Here's how the part is built. I have some questions about the finished solid (model axes, mm). A direction names the side the tool comes from. Give positions to 0.01 mm unless a question says otherwise; leave off trailing zeros. Loops run counter-clockwise (first coordinate to the right, second up) from the corner with the lowest first, then second, coordinate; pieces in that order, holes last.
Q1. If we section it at B-B (z = -24.5): Please give me the cut outline in (x, y).
Q2. I need wall thicknesses on line 1 (Y direction, x = -8.27, z = 0.2) (3 decimals); line 2 (Z direction, x = 1.5, y = 7.75); line 3 (Y direction, x = 0, z = -28.85). Which ranges of each line are inside material? Lowest first, please.
Q3. If we section it at D-D (x = -8.27): Please give me the cut outline in (y, z) (3 decimals), plus the area to 3 significant figures.
Q4. If we section it at A-A (x = 0): Please give me the cut outline in (y, z) (3 decimals).
Q5. For faces 1 (the face through (-12.84, 7.87, -29.26)), 2 (the face through (17, -2, -27)), 3 (the face through (0, 5.4, -33)), which set-ups out of +Z, -Z, +X, -X, +Y, -Y let a thin tool reach every point of the face, with its end or its side?
Q6. Will these pins go through, and if not, where does the flat tip stop? P1, Ø5.5, axis at x = -0.5, z = -31.5, coming from the -Y side; P2, Ø2.5, axis at x = 17, z = -2.5, coming from the -Y side; P3, Ø1.6, axis at x = -9.5, z = -29.5, coming from the +Y side.
Q7. We'd pull the mould along Y, two halves only. Please class faces 4 (the face through (5.8, 3, -33)), 5 (the face through (4.13, 9.16, -29.26)), 6 (the face through (17, -2, -2)), 7 (the face through (-9.788, 3.106, -29.26)): +Y half, -Y half, draft (parallel to the pull), parting line (faces both ways), or undercut.
from build123d import *

# Parameters (mm, degrees)
SKETCH_1_W          = 27
SKETCH_1_H          = 17
EXTRUDE_1_DEPTH     = 1
SKETCH_2_R          = 2.55
CUT_EXTRUDE_1_DEPTH = 16.984367363
EXTRUDE_2_DEPTH     = 17
SKETCH_6_W          = 1.5
SKETCH_6_H          = 2
EXTRUDE_3_DEPTH     = 2
CHAMFER_1_SIZE      = 1
CUT_EXTRUDE_4_REACH = 39.316
SKETCH_8_R          = 2
FILLET_1_R          = 3
SKETCH_9_W          = 7
SKETCH_9_H          = 13
EXTRUDE_4_DEPTH     = 1.5
SKETCH_7_R          = 1.35
CUT_EXTRUDE_5_DEPTH = 10
CUT_EXTRUDE_6_REACH = 41.373
FILLET_2_R          = 2.2
SKETCH_13_W         = 11.6
SKETCH_13_H         = 5.4
EXTRUDE_6_DEPTH     = 5.4


with BuildPart() as part:
    # 草图1 → 凸台-拉伸1 (new body)
    with BuildSketch(Plane.XY):
        Rectangle(SKETCH_1_W, SKETCH_1_H)
    extrude(amount=EXTRUDE_1_DEPTH)

    # 草图2 → 切除-拉伸1 (cut, through all)
    with BuildSketch(Plane.XY.offset(1)):
        with Locations((0, 4.125)):
            Circle(SKETCH_2_R)
        with Locations((0, -4.125)):
            Circle(SKETCH_2_R)
        with Locations((8.27, 4.125)):
            Circle(SKETCH_2_R)
        with Locations((8.27, -4.125)):
            Circle(SKETCH_2_R)
        with Locations((-8.27, 4.125)):
            Circle(SKETCH_2_R)
        with Locations((-8.27, -4.125)):
            Circle(SKETCH_2_R)
    extrude(amount=-CUT_EXTRUDE_1_DEPTH, mode=Mode.SUBTRACT)

    # 草图3 → 凸台-拉伸2 (add)
    with BuildSketch(Plane.XZ.offset(8.5)):
        Polygon((13.5, 0), (19, 0), (19, -28.5), (-13.5, -28.5), (-13.5, -30), (20.5, -30), (20.5, 1), (13.5, 1), align=None)
    extrude(amount=-EXTRUDE_2_DEPTH)

    # 草图6 → 凸台-拉伸3 (add, symmetric)
    with BuildSketch(Plane(origin=(0, 0, 0), x_dir=(1, 0, 0), z_dir=(0, 1, 0))):
        Polygon((19, 0), (19, 5), (14, 0), align=None)
        Polygon((19, 28.5), (14, 28.5), (19, 23.5), align=None)
        with Locations((18.25, 20)):
            Rectangle(SKETCH_6_W, SKETCH_6_H)
    extrude(amount=EXTRUDE_3_DEPTH, both=True)

    # 倒角1
    chamfer_1_edges = [part.edges().sort_by_distance(p)[0] for p in [
        (-13.5, 0, 0),
    ]]
    chamfer(chamfer_1_edges, length=CHAMFER_1_SIZE - 0.0001)  # a hair under: the kernel refuses the full size

    # 草图8 → 切除-拉伸4 (cut, up to next)
    with BuildSketch(Plane(origin=(0, 0, 0), x_dir=(-1, 0, 0), z_dir=(0, 0, -1)), mode=Mode.PRIVATE) as cut_extrude_4_sk1:
        Circle(SKETCH_8_R)
    cut_extrude_4_tool1 = extrude(cut_extrude_4_sk1.sketch, amount=-CUT_EXTRUDE_4_REACH, mode=Mode.PRIVATE) & part.part
    add(cut_extrude_4_tool1.solids().sort_by_distance((0, 0, 0))[0], mode=Mode.SUBTRACT)

    # 圆角1
    fillet_1_edges = [part.edges().sort_by_distance(p)[0] for p in [
        (20.5, 0, 1),
        (20.5, 0, -30),
        (19, 5.25, -28.5),
        (19, 5.25, 0),
        (19, -5.25, 0),
        (19, -5.25, -28.5),
    ]]
    fillet(fillet_1_edges, radius=FILLET_1_R)

    # 草图9 → 凸台-拉伸4 (add)
    with BuildSketch(Plane(origin=(0, 0, -30), x_dir=(-1, 0, 0), z_dir=(0, 0, -1))):
        with Locations((0, 6.5)):
            Rectangle(SKETCH_9_W, SKETCH_9_H)
    extrude(amount=-EXTRUDE_4_DEPTH)

    # 草图7 → 切除-拉伸5 (cut)
    with BuildSketch(Plane(origin=(0, 0, -30), x_dir=(-1, 0, 0), z_dir=(0, 0, -1))):
        with Locations((0, 10)):
            Circle(SKETCH_7_R)
        with Locations((-8.5, 2.7)):
            Circle(SKETCH_7_R)
        with Locations((8.5, 2.7)):
            Circle(SKETCH_7_R)
    extrude(amount=-CUT_EXTRUDE_5_DEPTH, mode=Mode.SUBTRACT)

    # 草图11 → 切除-拉伸6 (cut, up to next)
    with BuildSketch(Plane(origin=(0, 0, -30), x_dir=(-1, 0, 0), z_dir=(0, 0, -1)), mode=Mode.PRIVATE) as cut_extrude_6_sk1:
        with BuildLine():
            Line((13.5, -8.5), (13.5, 0))
            Line((13.5, 0), (-9, 0))
            ThreePointArc((-9, 0), (-15.01040764, -2.48959236), (-17.5, -8.5))
            Line((-17.5, -8.5), (13.5, -8.5))
        make_face()
    cut_extrude_6_tool1 = extrude(cut_extrude_6_sk1.sketch, amount=-CUT_EXTRUDE_6_REACH, mode=Mode.PRIVATE) & part.part
    add(cut_extrude_6_tool1.solids().sort_by_distance((1.149624, -4.397011, -30))[0], mode=Mode.SUBTRACT)

    # 圆角2
    fillet_2_edges = [part.edges().sort_by_distance(p)[0] for p in [
        (-3.5, 13, -29.25),
        (-3.5, 8.5, -29.25),
        (3.5, 13, -29.25),
        (3.5, 8.5, -29.25),
        (-13.5, 0, -29.25),
        (-13.5, 8.5, -29.25),
    ]]
    fillet(fillet_2_edges, radius=FILLET_2_R)

    # 草图13 → 凸台-拉伸6 (add)
    with BuildSketch(Plane(origin=(0, 0, -30), x_dir=(-1, 0, 0), z_dir=(0, 0, -1))):
        with Locations((0, 2.7)):
            Rectangle(SKETCH_13_W, SKETCH_13_H)
    extrude(amount=EXTRUDE_6_DEPTH)


solid = part.part
Check sheet entries:
1. outline: (18, -2) - (19, -2) - (19, -8.5) - (20.5, -8.5) - (20.5, 8.5) - (19, 8.5) - (19, 2) - (18, 2) - close
2. line 1: y = -8.5 to -6.675, -1.575 to 1.575, 6.675 to 8.5
2. line 2: z = -30 to -28.5, 0 to 1
2. line 3: y = 0 to 8.65, 11.35 to 13
3. outline: (-8.5, 0) - (-6.675, 0) - (-6.675, 1) - (-8.5, 1) - close; (-1.575, 0) - (1.575, 0) - (1.575, 1) - (-1.575, 1) - close; (0, -30) - (1.37, -30) - (1.37, -28.5) - (0, -28.5) - close; (4.03, -30) - (8.5, -30) - (8.5, -28.5) - (4.03, -28.5) - close; (6.675, 0) - (8.5, 0) - (8.5, 1) - (6.675, 1) - close
3. area: 15.6 mm2
4. outline: (-8.5, 0) - (-6.675, 0) - (-6.675, 1) - (-8.5, 1) - close; (0, -35.4) - (5.4, -35.4) - (5.4, -30) - (8.65, -30) - (8.65, -28.5) - (0, -28.5) - close; (6.675, 0) - (8.5, 0) - (8.5, 1) - (6.675, 1) - close; (11.35, -30) - (13, -30) - (13, -28.5) - (11.35, -28.5) - close
5. face 1: -Z, -X, +Y
5. face 2: -X, -Y
5. face 3: -Z, +X, -X, +Y
6. P1: stops at y = 0
6. P2: stops at y = -2
6. P3: stops at y = 8.5
7. face 4: draft
7. face 5: +Y half
7. face 6: -Y half
7. face 7: undercut
